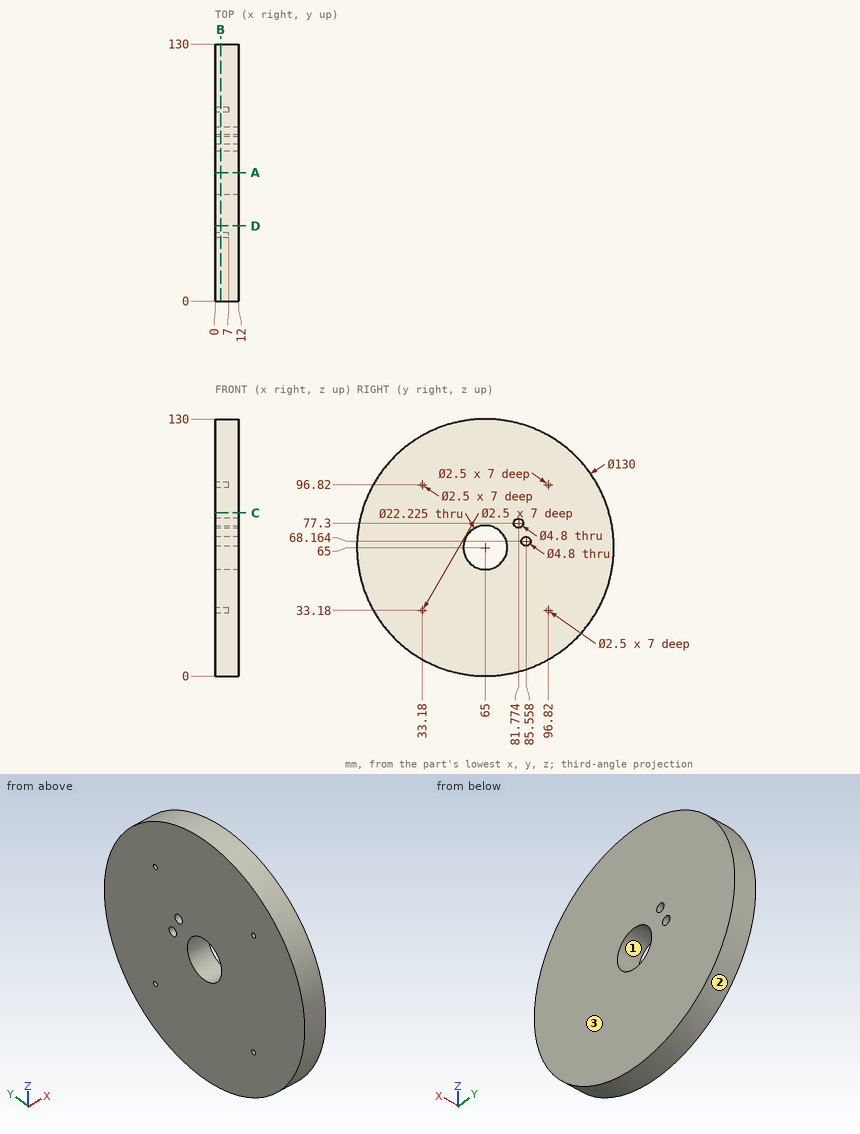
Print and shaded views of the part. All mm, measured from the part's lowest x, y and z. Give positions to 0.01 mm unless a question says otherwise; leave off trailing zeros. Loops run counter-clockwise (first coordinate to the right, second up) from the corner with the lowest first, then second, coordinate; pieces in that order, holes last.
1) Wall check: line 1 (Y direction, x = 5.5, z = 65); line 2 (Z direction, x = 3.25, y = 33) (1 decimal); line 3 (Z direction, x = 7.75, y = 69). Give the ranges that are in metal, low to high.
2) Saw through at D-D (y = 38). Write the cut outline in (x, z), plus the area to 3 significant figures.
3) Saw through at C-C (z = 82.5). Write the cut outline in (x, y).
4) Saw through at A-A (y = 65). Write the cut outline in (x, z).
5) Pull direction Y, two halves, no side cores. Call the marked faces 1, 2 and 3: +Y half, -Y half, draft (parallel to the pull), parting line (faces both ways), or undercut.
6) Saw through at B-B (x = 2.75). Count the separate pieces of the cut face and the enclosed holes in it, plus the area to 3 significant figures.
7) Flat gauge pins, fed straight in: pin 1 Ø0.8 at (y, z) = (96.5, 33.5) entering from -X; pin 2 Ø2 at (x, y) = (9.5, 89.5) entering from -Z; pin 3 Ø5 at (x, z) = (4.5, 32.5) entering from -Y. Where does each tip first touch, or does it go through?
Answer block:
1. line 1: y = 0 to 53.89, 76.11 to 130
1. line 2: z = 8.4 to 31.9, 34.4 to 95.6, 98.1 to 121.6
1. line 3: z = 0.12 to 54.63, 75.37 to 129.88
2. outline: (0, 5.87) - (12, 5.87) - (12, 124.13) - (0, 124.13) - close
2. area: 1,420 mm2
3. outline: (0, 2.4) - (12, 2.4) - (12, 127.6) - (0, 127.6) - close
4. outline: (0, 0) - (12, 0) - (12, 53.89) - (0, 53.89) - close; (0, 76.11) - (12, 76.11) - (12, 130) - (0, 130) - close
5. face 1: undercut
5. face 2: parting line
5. face 3: draft
6. separate pieces: 1
6. enclosed holes: 7
6. area: 12,800 mm2
7. pin 1: stops at x = 7
7. pin 2: stops at z = 4.4
7. pin 3: stops at y = 7.34
